from build123d import *

# Parameters (mm, degrees)
SKETCH1_W           = 25
SKETCH1_H           = 10
SKETCH1_R           = 1.05
BOSS_EXTRUDE1_DEPTH = 3
SKETCH3_W           = 8
SKETCH3_H           = 13
BOSS_EXTRUDE2_DEPTH = 10
SKETCH4_R           = 0.7
CUT_EXTRUDE1_DEPTH  = 21.621590627
SKETCH5_R           = 0.95
CUT_EXTRUDE2_DEPTH  = 3.5
CHAMFER1_SIZE       = 3


with BuildPart() as part:
    # Sketch1 → Boss-Extrude1 (new body)
    with BuildSketch(Plane(origin=(0, 0, 0), x_dir=(1, 0, 0), z_dir=(0, 1, 0))):
        Rectangle(SKETCH1_W, SKETCH1_H)
        with Locations(Location((-10, 2.5, 0), (0, 0, 270))):
            Circle(SKETCH1_R, mode=Mode.SUBTRACT)
        with Locations(Location((-10, -2.5, 0), (0, 0, 270))):
            Circle(SKETCH1_R, mode=Mode.SUBTRACT)
        with Locations(Location((10, 2.5, 0), (0, 0, 270))):
            Circle(SKETCH1_R, mode=Mode.SUBTRACT)
        with Locations(Location((10, -2.5, 0), (0, 0, 270))):
            Circle(SKETCH1_R, mode=Mode.SUBTRACT)
    extrude(amount=BOSS_EXTRUDE1_DEPTH)

    # Sketch3 → Boss-Extrude2 (add)
    with BuildSketch(Plane(origin=(0, 0, -5), x_dir=(-1, 0, 0), z_dir=(0, 0, -1))):
        with Locations((0, 6.5)):
            Rectangle(SKETCH3_W, SKETCH3_H)
    extrude(amount=-BOSS_EXTRUDE2_DEPTH)

    # Sketch4 → Cut-Extrude1 (cut, through all)
    with BuildSketch(Plane(origin=(0, 0, -5), x_dir=(-1, 0, 0), z_dir=(0, 0, -1))):
        with Locations((0, 9)):
            Circle(SKETCH4_R)
    extrude(amount=-CUT_EXTRUDE1_DEPTH, mode=Mode.SUBTRACT)

    # Sketch5 → Cut-Extrude2 (cut)
    with BuildSketch(Plane(origin=(0, 13, 0), x_dir=(1, 0, 0), z_dir=(0, 1, 0))):
        with Locations(Location((0, 3, 0), (0, 0, 180))):
            Circle(SKETCH5_R)
        with Locations(Location((0, -3, 0), (0, 0, 180))):
            Circle(SKETCH5_R)
    extrude(amount=-CUT_EXTRUDE2_DEPTH, mode=Mode.SUBTRACT)

    # Chamfer1
    chamfer1_edges = [part.edges().sort_by_distance(p)[0] for p in [
        (4, 3, 0),
        (-4, 3, 0),
    ]]
    chamfer(chamfer1_edges, length=CHAMFER1_SIZE)


solid = part.part
Could you check a few things on this model? Use its own coordinates, in mm. A direction names the side the tool comes from. Give positions to 0.01 mm unless a question says otherwise; leave off trailing zeros. Write each loop counter-clockwise with the first axis right and the second up, starting at its lowest first coordinate (ties: lowest second). Pieces come first, ordered by that corner, then holes. Notation, with made-up numbers: (35, 35.5) -> (71, 35.5) arc R13 ccw to (71, 45.5) -> close; hole circle Ø11 at (32, 68). An arc over 180 degrees is marked (long way). Answer as CSV lines item,"result". Start each with the question number.
(1) If we section it at A-A, the plane x = -10: Write out the boundary of the cut face in (y, z).
(2) If we section it at B-B, the plane y = 9: Write out the boundary of the cut face in (x, z), and give its area (3 significant figures).
(3) I'm going to push flat-ended pins straight in: pin 1 Ø2 at (y, z) = (11, -1) entering from -X; pin 2 Ø6 at (x, z) = (9.5, 1) entering from +Y; pin 3 Ø2 at (y, z) = (9.5, -1) entering from +X. Where does each tip first touch, or does it pass through?
(4) If we mould it in two halves opening along Z, with no side actions, what happens to faces 4 (the face through (10.89, 1.48, 3.06)), 5 (the face through (0, 13, 0)), 6 (the face through (0, 5, 5)), 7 (the face through (10.89, 1.48, -1.94))? For each: +Z half, -Z half, draft (parallel to the pull), parting line (faces both ways), or undercut.
(5) Which directions (+Z, -Z, +X, -X, +Y, -Y) give clear straight access to the entire face, cutting with the end or side of a thin tool? Please do faces 1 (the face through (-4, 9, 0)), 2 (the face through (10, 3, 0)), 3 (the face through (-0.51, 11.27, -2.2)).
(6) Please list where these lines run through material, in increasing order: line 1 (X direction, y = 1.55, z = 2.5); line 2 (X direction, y = 11.75, z = 3); line 3 (X direction, y = 9.25, z = 2).
(7) If we section it at D-D, the plane y = 2.75: Write out the boundary of the cut face in (x, z).
(8) If we section it at C-C, the plane x = 0: Write out the boundary of the cut face in (y, z), and give its area (3 significant figures).
Answer list:
1,outline,"(0, -5) -> (3, -5) -> (3, -3.55) -> (0, -3.55) -> close; (0, -1.45) -> (3, -1.45) -> (3, 1.45) -> (0, 1.45) -> close; (0, 3.55) -> (3, 3.55) -> (3, 5) -> (0, 5) -> close"
2,outline,"(-4, -5) -> (-0.7, -5) -> (-0.7, 5) -> (-4, 5) -> close; (0.7, -5) -> (4, -5) -> (4, 5) -> (0.7, 5) -> close"
2,area,"66.0 mm^2"
3,pin 1,"x = -4"
3,pin 2,"y = 3.5"
3,pin 3,"x = 4"
4,face 4,"undercut"
4,face 5,"draft"
4,face 6,"+Z half"
4,face 7,"undercut"
5,face 1,"+Z, -Z, -X, +Y"
5,face 2,"+Z, -Z, +X, +Y"
5,face 3,"+Y"
6,line 1,"-12.5 to -11.05, -8.95 to 8.95, 11.05 to 12.5"
6,line 2,"-4 to -0.95, 0.95 to 4"
6,line 3,"-4 to -0.65, 0.65 to 4"
7,outline,"(-12.5, -5) -> (12.5, -5) -> (12.5, 5) -> (-12.5, 5) -> close; hole circle Ø2.1 at (-10, -2.5); hole circle Ø2.1 at (-10, 2.5); hole circle Ø2.1 at (10, -2.5); hole circle Ø2.1 at (10, 2.5)"
8,outline,"(0, -5) -> (8.3, -5) -> (8.3, 5) -> (0, 5) -> close; (9.7, -5) -> (13, -5) -> (13, -3.95) -> (9.7, -3.95) -> close; (9.7, -2.05) -> (13, -2.05) -> (13, 2.05) -> (9.7, 2.05) -> close; (9.7, 3.95) -> (13, 3.95) -> (13, 5) -> (9.7, 5) -> close"
8,area,"103 mm^2"
